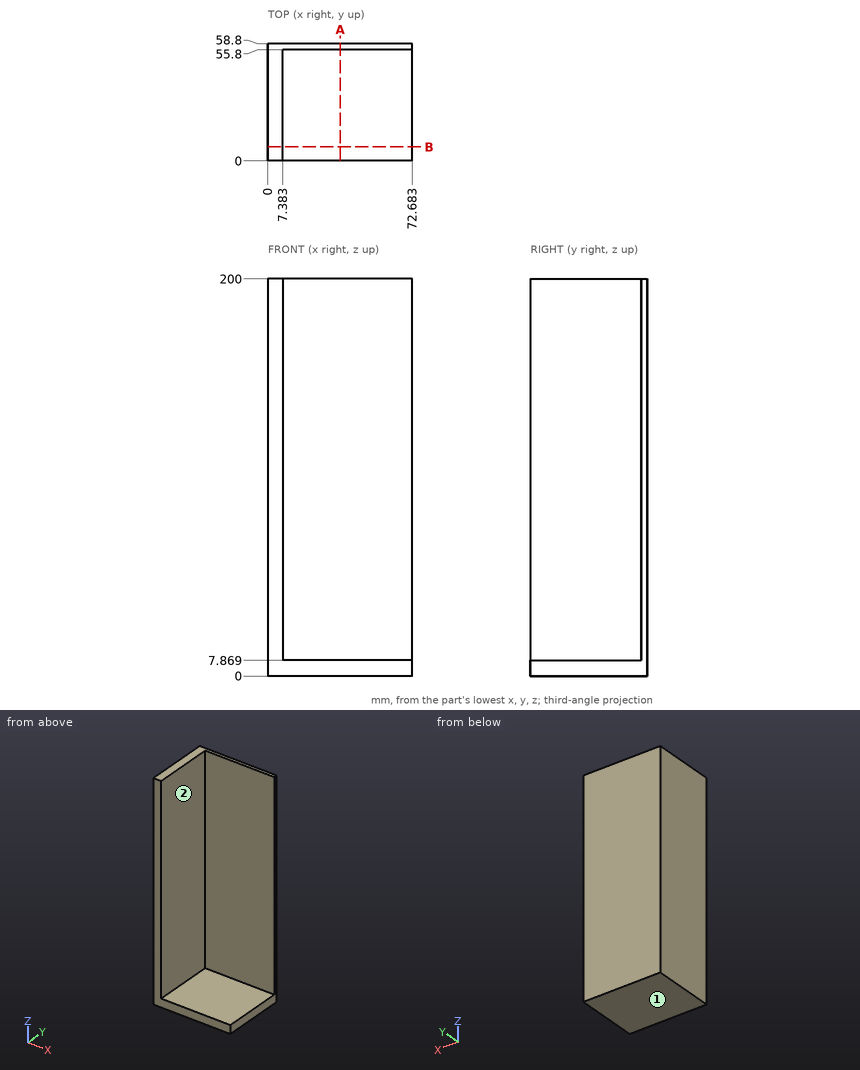
Verification items for this drawing (mm, ordinates from the low corner). A direction names the side the tool comes from. Coordinates: 2 decimals unless noted, no trailing zeros. Order: outer loops, then holes, each group sorted by start corner. A loop starts at its lowest first (then second) coordinate and runs counter-clockwise, first axis right, second up. Notation, with made-up numbers: (87, -0.75) -> (118, -0.75) arc R17 cw to (118, 17.25) -> close; hole circle Ø4 at (79.25, -11.75). An arc over 180 degrees is marked (long way). Answer as CSV lines item,"result". Start each with the question number.
1) Cross-section at B-B, the plane y = 7. Record the boundary of the cut face in (x, z), then the cut area to 3 significant figures.
2) Gauge pin test, flat ends, axial feed: pin 1 Ø8 at (y, z) = (18, 69.5) entering from +X; pin 2 Ø5 at (x, z) = (11.5, 52) entering from -Y; pin 3 Ø10 at (x, y) = (16.5, 10) entering from +Z. Record the tip position at first contact, or that the pin passes through.
3) Set-up check for the marked faces 1 and 2: record each of +Z, -Z, +X, -X, +Y, -Y from which the full face is reachable in a straight line by a thin tool's end or side.
4) Cross-section at A-A, the plane x = 36.5. Record the boundary of the cut face in (y, z).
5) Material ranges on L1, parallel to Y at x = 16, z = 46.5; L2, parallel to Z at x = 69.5, y = 6; L3, parallel to X at y = 8, z = 42.5, recorded low to high. Write a range as [from, to].
Conclusion:
1,outline,"(0, 0) -> (72.68, 0) -> (72.68, 7.87) -> (7.38, 7.87) -> (7.38, 200) -> (0, 200) -> close"
1,area,"1,990 mm²"
2,pin 1,"stops at x = 7.38"
2,pin 2,"stops at y = 55.8"
2,pin 3,"stops at z = 7.87"
3,face 1,"-Z, +X, -X, +Y, -Y"
3,face 2,"+Z, +X, -Y"
4,outline,"(0, 0) -> (58.8, 0) -> (58.8, 200) -> (55.8, 200) -> (55.8, 7.87) -> (0, 7.87) -> close"
5,L1,"y = [55.8, 58.8]"
5,L2,"z = [0, 7.87]"
5,L3,"x = [0, 7.38]"
